from build123d import *

# Parameters (mm, degrees)
SKETCH_W        = 76.2
SKETCH_H        = 34
PAD_DEPTH       = 3
SKETCH001_R     = 2.25
POCKET_DEPTH    = 3.001
SKETCH002_W     = 76.2
SKETCH002_H     = 5
PAD001_DEPTH    = 37
POCKET001_DEPTH = 34.001
SKETCH004_W     = 25
SKETCH004_H     = 37
SKETCH004_W_2   = 9
POCKET002_DEPTH = 34.001
FILLET_R        = 10
FILLET001_R     = 5
FILLET002_R     = 3
PAD002_DEPTH    = 21
SKETCH005_W     = 19.546381
SKETCH005_H     = 5.254696
POCKET003_DEPTH = 3.001


with BuildPart() as part:
    # Sketch → Pad (new body)
    with BuildSketch(Plane.XY):
        Rectangle(SKETCH_W, SKETCH_H)
    extrude(amount=PAD_DEPTH)

    # Sketch001 (on Face6 of Pad) → Pocket (cut, through all)
    with BuildSketch(Plane.XY.offset(3)):
        with Locations((-30.1, 9)):
            Circle(SKETCH001_R)
        with Locations((30.1, 9)):
            Circle(SKETCH001_R)
    extrude(amount=-POCKET_DEPTH, mode=Mode.SUBTRACT)

    # Sketch002 (on Face5 of Pocket) → Pad001 (join)
    with BuildSketch(Plane.XY.offset(3)):
        with Locations((0, -14.5)):
            Rectangle(SKETCH002_W, SKETCH002_H)
    extrude(amount=PAD001_DEPTH)

    # Sketch003 (on Face12 of Pad001) → Pocket001 (cut, through all)
    with BuildSketch(Plane.XZ.offset(17)):
        with BuildLine():
            ThreePointArc((-5.25, 16.5), (-3, 14.25), (-0.75, 16.5))
            Line((-0.75, 16.5), (-0.75, 36.5))
            ThreePointArc((-0.75, 36.5), (-3, 38.75), (-5.25, 36.5))
            Line((-5.25, 16.5), (-5.25, 36.5))
        make_face()
        with BuildLine():
            ThreePointArc((17.25, 7), (19.5, 4.75), (21.75, 7))
            Line((21.75, 7), (21.75, 27))
            ThreePointArc((21.75, 27), (19.5, 29.25), (17.25, 27))
            Line((17.25, 7), (17.25, 27))
        make_face()
    extrude(amount=-POCKET001_DEPTH, mode=Mode.SUBTRACT)

    # Sketch004 (on Face12 of Pocket001) → Pocket002 (cut, through all)
    with BuildSketch(Plane.XZ.offset(17)):
        with Locations((-25.6, 21.5)):
            Rectangle(SKETCH004_W, SKETCH004_H)
        with Locations((33.6, 21.5)):
            Rectangle(SKETCH004_W_2, SKETCH004_H)
    extrude(amount=-POCKET002_DEPTH, mode=Mode.SUBTRACT)

    # Fillet
    fillet_edges = [part.edges().sort_by_distance(p)[0] for p in [
        (-13.1, -14.5, 40),
        (29.1, -14.5, 40),
    ]]
    fillet(fillet_edges, radius=FILLET_R)

    # Fillet001
    fillet001_edges = [part.edges().sort_by_distance(p)[0] for p in [
        (-13.1, -14.5, 3),
        (29.1, -14.5, 3),
    ]]
    fillet(fillet001_edges, radius=FILLET001_R)

    # Fillet002
    fillet002_edges = [part.edges().sort_by_distance(p)[0] for p in [
        (8, -12, 3),
    ]]
    fillet(fillet002_edges, radius=FILLET002_R)

    # Fillet002 Face31 → Pad002 (add)
    with BuildSketch(Plane(origin=(0, -17, 1.5), x_dir=(-1, 0, 0), z_dir=(0, -1, 0))):
        Polygon((-38.1, -1.5), (-34.1, -1.5), (-29.1, -1.5), (13.1, -1.5), (18.1, -1.5), (38.1, -1.5), (38.1, 1.5), (-38.1, 1.5), align=None)
    extrude(amount=PAD002_DEPTH)

    # Sketch005 (on Face29 of Pad002) → Pocket003 (cut, through all)
    with BuildSketch(Plane.XY.offset(3)):
        with Locations((7.336419, -26.952593)):
            Rectangle(SKETCH005_W, SKETCH005_H)
    extrude(amount=-POCKET003_DEPTH, mode=Mode.SUBTRACT)


solid = part.part
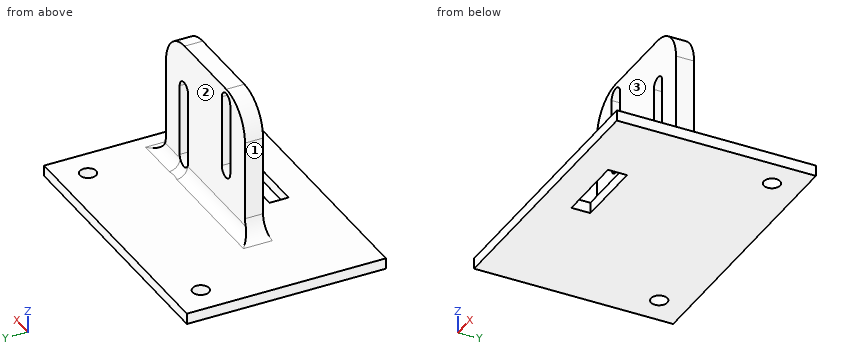
Source: CAD feature listing. Evaluate the final solid. Frame: model axes, mm. Face numbers are marked on the shaded views. A direction names the side the tool comes from. Coordinates: 2 decimals unless noted, no trailing zeros. Loops run counter-clockwise (first coordinate to the right, second up) from the corner with the lowest first, then second, coordinate; pieces in that order, holes last. Notation, with made-up numbers: M 35.25,-35 L 79.25,-35 A31 ccw 79.25,0 Z; hole C 21,43 d1. An arc over 180 degrees is marked long. Answer in a Markdown table with one row per item.
Q1. First-contact query: pin 1 (5 mm diameter, centred on x = -3, z = 25, fed in from +Y); pin 2 (3 mm diameter, centred on x = 21, z = 25, fed in from -Y); pin 3 (2.5 mm diameter, centred on y = -15, z = 15.5, fed in from -X); pin 4 (10 mm diameter, centred on x = 14, y = 2.5, fed in from -Z). Flat tips, straight axial feed; report the tip coordinate or a pass-through.
Answers below:
| item | result |
|---|---|
| pin 1 | stops at y = -12 |
| pin 2 | stops at y = -17 |
| pin 3 | stops at x = -13.1 |
| pin 4 | stops at z = 0 |
Q2. Section C-C on y = 8. Return the cut outline in (x, z), plus the area to 3 significant figures.
Answers below:
| item | result |
|---|---|
| outline | M -38.1,0 L -32.12,0 L -32.12,3 L -38.1,3 Z; M -28.08,0 L 28.08,0 L 28.08,3 L -28.08,3 Z; M 32.12,0 L 38.1,0 L 38.1,3 L 32.12,3 Z |
| area | 204 mm^2 |
Q3. Section D-D on x = 15.5. Return the cut outline in (y, z).
Answers below:
| item | result |
|---|---|
| outline | M -38,0 L -29.58,0 L -29.58,3 L -38,3 Z; M -24.33,0 L 17,0 L 17,3 L -9,3 A3 cw -12,6 L -12,40 L -17,40 L -17,3 L -24.33,3 Z |
Q4. Set-up query: the marked faces 1, 2 and 3. Return all of +Z, -Z, +X, -X, +Y, -Y with unobstructed straight access to the full face (end or side cutting, diameter ignored); none if empty.
Answers below:
| item | result |
|---|---|
| face 1 | +Z, -X, +Y, -Y |
| face 2 | +Z, +X, -X, +Y |
| face 3 | +Z, +X, -X, -Y |
Q5. Ray query, probe 1 along Y at (x, z) = (-30.1, 1.4); probe 2 along X at (y, z) = (-13, 30); probe 3 along Z at (x, y) = (-28.5, -19). Return the intervals inside material, ascending. Write a range as from..to.
Answers below:
| item | result |
|---|---|
| probe 1 | y = -38..6.75, 11.25..17 |
| probe 2 | x = -13.1..-5.25, -0.75..29.1 |
| probe 3 | z = 0..3 |
Q6. Section A-A on x = -30.1. Return the cut outline in (y, z).
Answers below:
| item | result |
|---|---|
| outline | M -38,0 L 6.75,0 L 6.75,3 L -38,3 Z; M 11.25,0 L 17,0 L 17,3 L 11.25,3 Z |
Q7. Section B-B on z = 25.5. Return the cut outline in (x, y), plus the area to 3 significant figures.
Answers below:
| item | result |
|---|---|
| outline | M -13.1,-17 L -5.25,-17 L -5.25,-12 L -13.1,-12 Z; M -0.75,-17 L 17.25,-17 L 17.25,-12 L -0.75,-12 Z; M 21.75,-17 L 29.1,-17 L 29.1,-12 L 21.75,-12 Z |
| area | 166 mm^2 |
